Can you work these out from the model? Positions are in its coordinate system, mm. A direction names the side the tool comes from. Round coordinates to 2 decimals unless told otherwise and drop trailing zeros. Loops run counter-clockwise (first coordinate to the right, second up) from the corner with the lowest first, then second, coordinate; pieces in that order, holes last.
from build123d import *

# Parameters (mm, degrees)
SKETCH1_W           = 160
SKETCH1_H           = 50.8
BOSS_EXTRUDE1_DEPTH = 10
SKETCH2_R           = 6.35
BOSS_EXTRUDE2_DEPTH = 160
SKETCH3_W           = 16
SKETCH3_H           = 40
CUT_EXTRUDE1_DEPTH  = 71
SKETCH5_R           = 3.9243
BOSS_EXTRUDE3_DEPTH = 10


with BuildPart() as part:
    # Sketch1 → Boss-Extrude1 (new body)
    with BuildSketch(Plane(origin=(0, 0, 0), x_dir=(1, 0, 0), z_dir=(0, 1, 0))):
        with Locations((80, 25.4)):
            Rectangle(SKETCH1_W, SKETCH1_H)
    extrude(amount=BOSS_EXTRUDE1_DEPTH)

    # Sketch2 → Boss-Extrude2 (add, through all)
    with BuildSketch(Plane.ZY):
        with BuildLine():
            Line((-50.8, 10), (-39.444175854, 40.268882668))
            ThreePointArc((-39.444175854, 40.268882668), (-25.4, 50), (-11.355824146, 40.268882668))
            Line((-11.355824146, 40.268882668), (0, 10))
            Line((0, 10), (-50.8, 10))
        make_face()
        with Locations((-25.4, 35)):
            Circle(SKETCH2_R, mode=Mode.SUBTRACT)
    extrude(amount=-BOSS_EXTRUDE2_DEPTH)

    # Sketch3 → Cut-Extrude1 (cut)
    with BuildSketch(Plane(origin=(0, 0, -50.8), x_dir=(-1, 0, 0), z_dir=(0, 0, -1))):
        with Locations((-130, 30)):
            Rectangle(SKETCH3_W, SKETCH3_H)
        with Locations((-98, 30)):
            Rectangle(SKETCH3_W, SKETCH3_H)
        with Locations((-66, 30)):
            Rectangle(SKETCH3_W, SKETCH3_H)
        with Locations((-34, 30)):
            Rectangle(SKETCH3_W, SKETCH3_H)
    extrude(amount=-CUT_EXTRUDE1_DEPTH, mode=Mode.SUBTRACT)

    # Sketch5 → Boss-Extrude3 (add)
    # profile 1 of 2: a face of its own
    with BuildSketch(Plane.XZ):
        with BuildLine():
            Line((160, 0), (209.86380094, -8.4))
            ThreePointArc((209.86380094, -8.4), (224.239528875, -25.4), (209.86380094, -42.4))
            Line((209.86380094, -42.4), (160, -50.8))
            Line((160, -50.8), (160, 0))
        make_face()
        with Locations(Location((207, -25.4, 0), (0, 0, 90))):
            Circle(SKETCH5_R, mode=Mode.SUBTRACT)
    # profile 2 of 2: a face of its own
    with BuildSketch(Plane.XZ):
        with BuildLine():
            Line((0, 0), (-49.86380094, -8.4))
            ThreePointArc((-49.86380094, -8.4), (-64.239528875, -25.4), (-49.86380094, -42.4))
            Line((-49.86380094, -42.4), (0, -50.8))
            Line((0, -50.8), (0, 0))
        make_face()
        with Locations(Location((-47, -25.4, 0), (0, 0, 270))):
            Circle(SKETCH5_R, mode=Mode.SUBTRACT)
    extrude(amount=-BOSS_EXTRUDE3_DEPTH)


solid = part.part
(1) If we section it at D-D, the plane z = -25.4: State how many separate pieces and enclosed holes the cut face has, then the cut area to 3 significant figures.
Worked answers:
separate pieces: 8
enclosed holes: 0
area: 5,350 mm2
(2) Will these pins go through, and if not, where does the flat tip stop? P1, Ø8, axis at x = 30.5, z = -15.5, coming from the +Y side; P2, Ø3, axis at x = 9.5, z = -14, coming from the +Y side; P3, Ø7.5, axis at y = 35, z = -25.4, coming from the +X side; P4, Ø4, axis at x = 85.5, y = 33.5, coming from the +Z side.
Worked answers:
P1: stops at y = 10
P2: stops at y = 46.27
P3: passes through
P4: stops at z = -8.07
(3) For faces 5 (the flat face through (98, 10, -26)), 6 (the flat face through (185, 10, -25)), 7 (the flat face through (185.28, 4.93, -46.54)), which set-ups out of +Z, -Z, +X, -X, +Y, -Y let a thin tool reach every point of the face, with its end or its side?
Worked answers:
face 5: +Z, -Z, +Y
face 6: +Z, -Z, +X, +Y
face 7: -Z, +X, +Y, -Y
(4) If we section it at B-B, the plane x = -47: List the corners of the cut face in (y, z) for me.
Worked answers:
outline: (0, -42.88) - (10, -42.88) - (10, -29.32) - (0, -29.32) - close; (0, -21.48) - (10, -21.48) - (10, -7.92) - (0, -7.92) - close
(5) If we section it at C-C, the plane y = 22.5: List the corners of the cut face in (x, z) for me.
Worked answers:
outline: (0, -46.11) - (26, -46.11) - (26, -4.69) - (0, -4.69) - close; (42, -46.11) - (58, -46.11) - (58, -4.69) - (42, -4.69) - close; (74, -46.11) - (90, -46.11) - (90, -4.69) - (74, -4.69) - close; (106, -46.11) - (122, -46.11) - (122, -4.69) - (106, -4.69) - close; (138, -46.11) - (160, -46.11) - (160, -4.69) - (138, -4.69) - close
(6) If I drill on line 1 (X direction, y = 11, z = -28.5); line 2 (X direction, y = 9, z = -22.5); line 3 (Y direction, x = 80, z = -25.4), over which ranges is the centre line in solid material (lowest first)?
Worked answers:
line 1: x = 0 to 26, 42 to 58, 74 to 90, 106 to 122, 138 to 160
line 2: x = -63.99 to -49.64, -44.36 to 204.36, 209.64 to 223.99
line 3: y = 0 to 28.65, 41.35 to 50
(7) If we section it at A-A, the plane y = 7: List the corners of the cut face in (x, z) for me.
Worked answers:
outline: (-49.86, -42.4) - (0, -50.8) - (160, -50.8) - (209.86, -42.4) arc R17.24 ccw to (209.86, -8.4) - (160, 0) - (0, 0) - (-49.86, -8.4) arc R17.24 ccw to start; hole circle Ø7.85 at (-47, -25.4); hole circle Ø7.85 at (207, -25.4)
(8) If we mould it in two halves opening along X, with no side actions, what happens to faces 1 (the cylindrical face through (12.818, 49.998, -25.654)), 2 (the cylindrical face through (224.236, 4.93, -25.061)), 3 (the cylindrical face through (-64.236, 4.93, -25.061)), 4 (the cylindrical face through (-43.11, 4.93, -24.89))? For each: released by +X, released by -X, zero draft, split by the parting line, or undercut.
Worked answers:
face 1: zero draft
face 2: released by +X
face 3: released by -X
face 4: undercut
